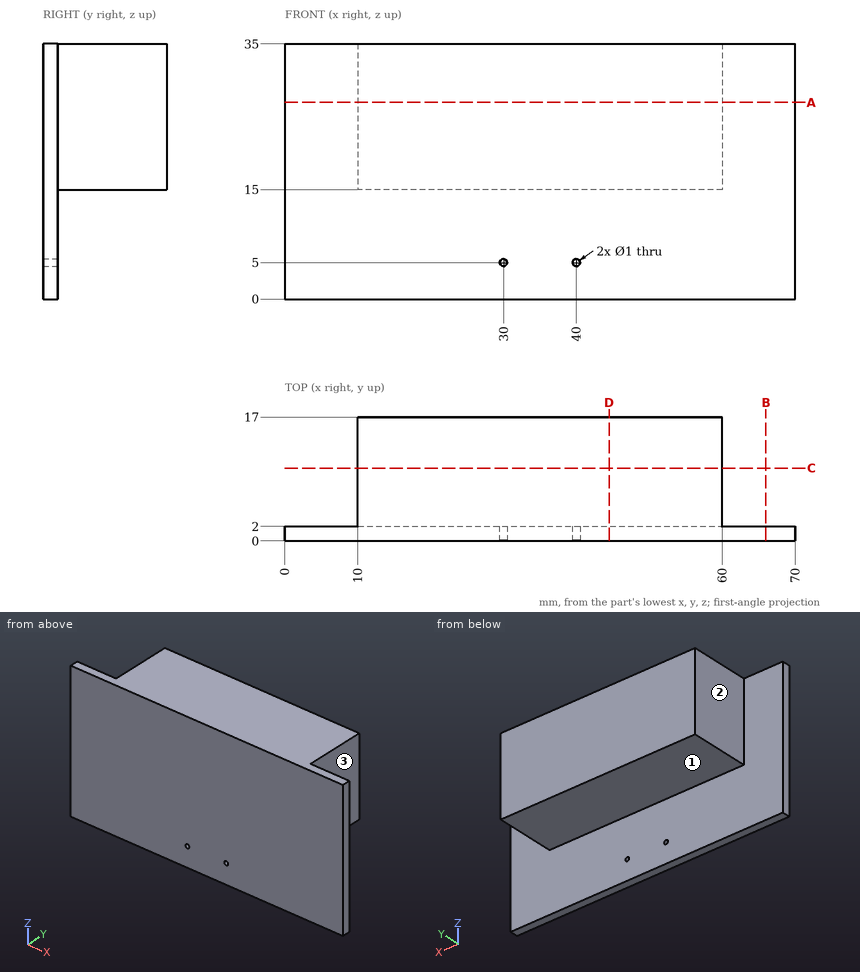
Check sheet for the drawn part. Datum: minimum x, y, z corner. Units: mm. A direction names the side the tool comes from. Coordinates: 2 decimals unless noted, no trailing zeros. Order: outer loops, then holes, each group sorted by start corner. A loop starts at its lowest first (then second) coordinate and runs counter-clockwise, first axis right, second up. Notation, with made-up numbers: M -33,61.25 L -8,61.25 A16 ccw -8,90.25 Z; hole C 20.5,27.25 d8. An arc over 180 degrees is marked long. One line per item, written item: value. Start each with the question number.
Item 1: Sectioned sample at C-C (y = 10). Enter the section's corners in (x, z), then the cut area to 3 significant figures.
Item 2: Sectioned sample at B-B (x = 66). Enter the section's corners in (y, z).
Item 3: Gauge pin test, flat ends, axial feed: pin 1 (4.5 mm diameter, centred on y = 6, z = 25, fed in from -X); pin 2 (8 mm diameter, centred on x = 47, y = 11, fed in from -Z); pin 3 (7.5 mm diameter, centred on y = 11, z = 28.5, fed in from +X). Record the tip position at first contact, or that the pin passes through.
Item 4: Sectioned sample at A-A (z = 27). Enter the section's corners in (x, y).
Item 5: Scan lines: probe 1 along X at (y, z) = (1.3, 5); probe 2 along Z at (x, y) = (30, 1.4); probe 3 along Y at (x, z) = (43, 10). Record each from-to range of solid material in increasing order.
Item 6: Access from +Z, -Z, +X, -X, +Y, -Y to the whole of each face (thin tool, end or side, straight path). Record for the marked faces 1, 2 and 3.
Item 7: Sectioned sample at D-D (x = 44.5). Enter the section's corners in (y, z).
Conclusion:
1. outline: M 10,15 L 60,15 L 60,35 L 10,35 Z
1. area: 1,000 mm^2
2. outline: M 0,0 L 2,0 L 2,35 L 0,35 Z
3. pin 1: stops at x = 10
3. pin 2: stops at z = 15
3. pin 3: stops at x = 60
4. outline: M 0,0 L 70,0 L 70,2 L 60,2 L 60,17 L 10,17 L 10,2 L 0,2 Z
5. probe 1: x = 0 to 29.5, 30.5 to 39.5, 40.5 to 70
5. probe 2: z = 0 to 4.5, 5.5 to 35
5. probe 3: y = 0 to 2
6. face 1: -Z, +X, -X, +Y
6. face 2: +Z, -Z, -X, +Y
6. face 3: +Z, -Z, +X, +Y
7. outline: M 0,0 L 2,0 L 2,15 L 17,15 L 17,35 L 0,35 Z
